from build123d import *

# Parameters (mm, degrees)
PLACA_START                   = -53.1
SK_PLACA_W                    = 70
SK_PLACA_H                    = 160
PLACA_DEPTH                   = 6.35
EXTREMOS_START                = -53.1
SK_EXTREMOS_R                 = 35
EXTREMOS_DEPTH                = 6.35
PASANTES_M4_SEPARADORES_START = -53.1
SK_PASANTES_M4_SEPARADORES_R  = 2.25
PASANTES_M4_SEPARADORES_DEPTH = 6.35
ALOJAMIENTO_696ZZ_START       = -51.75
SK_ALOJAMIENTO_696ZZ_R        = 7.475
ALOJAMIENTO_696ZZ_DEPTH       = 5
PASO_EXTRACTOR_START          = -53.1
SK_PASO_EXTRACTOR_R           = 4
PASO_EXTRACTOR_DEPTH          = 1.35
PASANTES_M4_EJEFALSO_J3_START = -53.1
SK_PASANTES_M4_EJEFALSO_J3_R  = 2.25
PASANTES_M4_EJEFALSO_J3_DEPTH = 6.35
SK_CAJAS_M4_SEPARADORES_R     = 4
CAJAS_M4_SEPARADORES_DEPTH    = 3.5


with BuildPart() as part:
    # Sk_Placa → Placa (new body)
    with BuildSketch(Plane(origin=(0, 0, 0), x_dir=(1, 0, 0), z_dir=(0, 1, 0)).offset(PLACA_START)):
        with Locations((0, -250)):
            Rectangle(SK_PLACA_W, SK_PLACA_H)
    extrude(amount=PLACA_DEPTH)

    # Sk_Extremos → Extremos (add)
    with BuildSketch(Plane(origin=(0, 0, 0), x_dir=(1, 0, 0), z_dir=(0, 1, 0)).offset(EXTREMOS_START)):
        with Locations((0, -170)):
            Circle(SK_EXTREMOS_R)
        with Locations((0, -330)):
            Circle(SK_EXTREMOS_R)
    extrude(amount=EXTREMOS_DEPTH)

    # Sk_Pasantes_M4_separadores → Pasantes_M4_separadores (cut)
    with BuildSketch(Plane(origin=(0, 0, 0), x_dir=(1, 0, 0), z_dir=(0, 1, 0)).offset(PASANTES_M4_SEPARADORES_START)):
        with Locations(Location((0, -250, 0), (0, 0, 270))):
            Circle(SK_PASANTES_M4_SEPARADORES_R)
        with Locations(Location((-22, -300, 0), (0, 0, 270))):
            Circle(SK_PASANTES_M4_SEPARADORES_R)
        with Locations(Location((22, -300, 0), (0, 0, 270))):
            Circle(SK_PASANTES_M4_SEPARADORES_R)
    extrude(amount=PASANTES_M4_SEPARADORES_DEPTH, mode=Mode.SUBTRACT)

    # Sk_Alojamiento_696ZZ → Alojamiento_696ZZ (cut)
    with BuildSketch(Plane(origin=(0, 0, 0), x_dir=(1, 0, 0), z_dir=(0, 1, 0)).offset(ALOJAMIENTO_696ZZ_START)):
        with Locations(Location((0, -170, 0), (0, 0, 270))):
            Circle(SK_ALOJAMIENTO_696ZZ_R)
    extrude(amount=ALOJAMIENTO_696ZZ_DEPTH, mode=Mode.SUBTRACT)

    # Sk_Paso_extractor → Paso_extractor (cut)
    with BuildSketch(Plane(origin=(0, 0, 0), x_dir=(1, 0, 0), z_dir=(0, 1, 0)).offset(PASO_EXTRACTOR_START)):
        with Locations(Location((0, -170, 0), (0, 0, 90))):
            Circle(SK_PASO_EXTRACTOR_R)
    extrude(amount=PASO_EXTRACTOR_DEPTH, mode=Mode.SUBTRACT)

    # Sk_Pasantes_M4_ejefalso_J3 → Pasantes_M4_ejefalso_J3 (cut)
    with BuildSketch(Plane(origin=(0, 0, 0), x_dir=(1, 0, 0), z_dir=(0, 1, 0)).offset(PASANTES_M4_EJEFALSO_J3_START)):
        with Locations(Location((0, -310.5, 0), (0, 0, 270))):
            Circle(SK_PASANTES_M4_EJEFALSO_J3_R)
        with Locations(Location((0, -349.5, 0), (0, 0, 270))):
            Circle(SK_PASANTES_M4_EJEFALSO_J3_R)
    extrude(amount=PASANTES_M4_EJEFALSO_J3_DEPTH, mode=Mode.SUBTRACT)

    # Sk_Cajas_M4_separadores → Cajas_M4_separadores (cut)
    with BuildSketch(Plane.XZ.offset(53.1)):
        with Locations(Location((0, 250, 0), (0, 0, 270))):
            Circle(SK_CAJAS_M4_SEPARADORES_R)
        with Locations(Location((22, 300, 0), (0, 0, 270))):
            Circle(SK_CAJAS_M4_SEPARADORES_R)
        with Locations(Location((-22, 300, 0), (0, 0, 270))):
            Circle(SK_CAJAS_M4_SEPARADORES_R)
    extrude(amount=-CAJAS_M4_SEPARADORES_DEPTH, mode=Mode.SUBTRACT)


solid = part.part
Can you work these out from the model? Positions are in its coordinate system, mm. A direction names the side the tool comes from. Coordinates: 2 decimals unless noted, no trailing zeros. Write each loop counter-clockwise with the first axis right and the second up, starting at its lowest first coordinate (ties: lowest second). Pieces come first, ordered by that corner, then holes. Notation, with made-up numbers: (26, 40.25) -> (66, 40.25) arc R10 ccw to (66, 51.25) -> close; hole circle Ø2 at (21, -23.75). An arc over 180 degrees is marked (long way). Write each question's results on one line, items separated by ' | '. Start each with the question number.
Item 1: If we section it at B-B, the plane y = -47.75: Write out the boundary of the cut face in (x, z) (3 decimals), and give its area (3 significant figures).
Item 2: If we section it at D-D, the plane x = -22: Write out the boundary of the cut face in (y, z), and give its area (3 significant figures).
Item 3: On a 3-axis mill with a long thin cutter (end or side, diameter ignored), from which of +Z, -Z, +X, -X, +Y, -Y can I reach the whole of each face in a straight line? I mean faces 5 (the cylindrical face through (0, -51, 254)), 6 (the cylindrical face through (0.099, -49.969, 347.252)), 7 (the flat face through (-3, -51.75, 173)). Say none if no direction works.
Item 4: I'm going to push flat-ended pins straight in: P1, Ø7, axis at x = 0, z = 250, coming from the -Y side; P2, Ø2, axis at x = -15.5, y = -48.5, coming from the +Z side; P3, Ø1, axis at x = -7, y = -47.5, coming from the +Z side; P4, Ø4, axis at x = 0, z = 310.5, coming from the -Y side. Where does each tip first touch, or does it pass through?
Item 5: Please list where these lines run through material, in increasing order: probe 1 along X at (y, z) = (-48.1, 300); probe 2 along Z at (x, y) = (-2, -47.5); probe 3 along Z at (x, y) = (19, -50).
Item 6: If we section it at A-A, the plane z = 250: Write out the boundary of the cut face in (x, y), and give its area (3 significant figures).
Item 7: Thinking about a two-plate mould opening in X: for faces 1 (the flat face through (35, -50, 251)), 2 (the flat face through (-35, -50, 251)), 3 (the flat face through (-24, -49.6, 298)), 4 (the cylindrical face through (22.099, -48.195, 297.752)), which applies, released by +X, released by -X, zero draft, split by the parting line, or undercut?
Item 8: If we section it at C-C, the plane z = 300: Write out the boundary of the cut face in (x, y), and give its area (3 significant figures).
Answer block:
1) outline: (-35, 170) arc R35 ccw to (35, 170) -> (35, 330) arc R35 ccw to (-35, 330) -> close; hole circle Ø4.5 at (-22, 300); hole circle Ø14.95 at (0, 170); hole circle Ø4.5 at (0, 250); hole circle Ø4.5 at (0, 310.5); hole circle Ø4.5 at (0, 349.5); hole circle Ø4.5 at (22, 300) | area: 14,800 mm²
2) outline: (-53.1, 142.78) -> (-46.75, 142.78) -> (-46.75, 297.75) -> (-49.6, 297.75) -> (-49.6, 296) -> (-53.1, 296) -> close; (-53.1, 304) -> (-49.6, 304) -> (-49.6, 302.25) -> (-46.75, 302.25) -> (-46.75, 357.22) -> (-53.1, 357.22) -> close | area: 1,320 mm²
3) face 5: -Y | face 6: +Y, -Y | face 7: +Y
4) P1: y = -49.6 | P2: z = 361.86 | P3: z = 364.39 | P4: through
5) probe 1: -35 to -24.25, -19.75 to 19.75, 24.25 to 35 | probe 2: 135.06 to 162.8, 177.2 to 248.97, 251.03 to 309.47, 311.53 to 348.47, 350.53 to 364.94 | probe 3: 140.61 to 297.35, 302.65 to 359.39
6) outline: (-35, -53.1) -> (-4, -53.1) -> (-4, -49.6) -> (-2.25, -49.6) -> (-2.25, -46.75) -> (-35, -46.75) -> close; (2.25, -49.6) -> (4, -49.6) -> (4, -53.1) -> (35, -53.1) -> (35, -46.75) -> (2.25, -46.75) -> close | area: 404 mm²
7) face 1: released by +X | face 2: released by -X | face 3: undercut | face 4: undercut
8) outline: (-35, -53.1) -> (-26, -53.1) -> (-26, -49.6) -> (-24.25, -49.6) -> (-24.25, -46.75) -> (-35, -46.75) -> close; (-19.75, -49.6) -> (-18, -49.6) -> (-18, -53.1) -> (18, -53.1) -> (18, -49.6) -> (19.75, -49.6) -> (19.75, -46.75) -> (-19.75, -46.75) -> close; (24.25, -49.6) -> (26, -49.6) -> (26, -53.1) -> (35, -53.1) -> (35, -46.75) -> (24.25, -46.75) -> close | area: 363 mm²
